Read the model definition and answer for the solid it produces. Units are mm, in the model's axes. A direction names the side the tool comes from. Give positions to 0.01 mm unless a question says otherwise; leave off trailing zeros. Order: outer loops, then holes, each group sorted by start corner. A loop starts at its lowest first (then second) coordinate and runs counter-clockwise, first axis right, second up. Notation, with made-up numbers: M -3.5,-30.5 L 54.5,-30.5 A27 ccw 54.5,-10.5 Z; hole C -25.75,16 d11. An arc over 180 degrees is marked long. One line per item, written item: value. Start each with the question number.
from build123d import *

# Parameters (mm, degrees)
PAD_DEPTH    = 6
POCKET_DEPTH = 5


with BuildPart() as part:
    # Sketch004 → Pad (new body)
    with BuildSketch(Plane.XY):
        with BuildLine():
            Line((-34.247254, 29.142098), (-34.247254, -40.731934))
            ThreePointArc((-34.247254, -40.731934), (-31.611215, -47.095895), (-25.247254, -49.731934))
            Line((-25.247254, -49.731934), (26.073956, -49.731934))
            ThreePointArc((26.073956, -49.731934), (31.73081, -47.388788), (34.073956, -41.731934))
            Line((34.073956, -41.731934), (34.073956, 29.142098))
            ThreePointArc((34.073956, 29.142098), (31.73081, 34.798952), (26.073956, 37.142098))
            Line((26.073956, 37.142098), (-26.247254, 37.142098))
            ThreePointArc((-26.247254, 37.142098), (-31.904109, 34.798952), (-34.247254, 29.142098))
        make_face()
    extrude(amount=PAD_DEPTH)

    # Sketch → Pocket (cut)
    with BuildSketch(Plane.XY.offset(6)):
        with BuildLine():
            ThreePointArc((0.2524, -41.074003), (14.410312, -36.50526), (22.890576, -24.282125))
            ThreePointArc((22.890576, -24.282125), (25.200826, -12.310293), (25.333783, -0.118314))
            ThreePointArc((25.333783, -0.118314), (22.825754, 10.910473), (17.275703, 20.765487))
            ThreePointArc((17.275703, 20.765487), (9.874199, 26.772272), (0.569118, 28.840892))
            ThreePointArc((0.55, 28.840771), (0.559559, 28.840801), (0.569118, 28.840892))
            Line((0.55, 28.840771), (0, 28.840771))
            Line((-0.55, 28.840771), (0, 28.840771))
            ThreePointArc((-0.569118, 28.840892), (-0.559559, 28.840801), (-0.55, 28.840771))
            ThreePointArc((-0.569118, 28.840892), (-9.874199, 26.772272), (-17.275703, 20.765487))
            ThreePointArc((-17.275703, 20.765487), (-22.825754, 10.910473), (-25.333783, -0.118314))
            ThreePointArc((-25.333783, -0.118314), (-25.200826, -12.310293), (-22.890576, -24.282125))
            ThreePointArc((-22.890576, -24.282125), (-14.410312, -36.50526), (-0.2524, -41.074003))
            ThreePointArc((-0.231547, -41.073858), (-0.241974, -41.073894), (-0.2524, -41.074003))
            Line((-0.231547, -41.073858), (0, -41.073858))
            Line((0.231547, -41.073858), (0, -41.073858))
            ThreePointArc((0.2524, -41.074003), (0.241974, -41.073894), (0.231547, -41.073858))
        make_face()
    extrude(amount=-POCKET_DEPTH, mode=Mode.SUBTRACT)


solid = part.part
Q1. Consider probe 1 along Z at (x, y) = (7, -39.5); probe 2 along X at (y, z) = (8, 5.6); probe 3 along Y at (x, z) = (9, 4.05). Determine where each line is inside the solid, lowest interval first.
Q2. Find section B-B, the plane y = -20. Give the vertices of the cut face in (x, z), then the cut area to 3 significant figures.
Q3. Determine the mould class of faces 3 (the cylindrical face through (-31.681, -47.026, 2.958)), 4 (the cylindrical face through (25.183, -12.48, 3.535)), 5 (the flat face through (-34.247, -5, 3)) for opening direction Y: released by +Y, released by -Y, zero draft, split by the parting line, or undercut.
Q4. Each of these flat-tipped pins is pushed along its axis until it touches: pin 1 (15.5 mm diameter, centred on x = 10.5, y = -4.5, fed in from +Z); pin 2 (5 mm diameter, centred on x = 18, y = -17.5, fed in from -Z). Where does it stop, or does it pass through?
Q5. Find section D-D, the plane y = 32. Give the vertices of the cut face in (x, z).
Q6. Find section C-C, the plane x = 2.5. Give the vertices of the cut face in (y, z).
Q7. A tool of negligible diameter and unlimited length cuts with its end or side. For faces 1 (the cylindrical face through (-22.768, 11.059, 3.535)), 2 (the flat face through (-23, 14, 6)), from which of +Z, -Z, +X, -X, +Y, -Y can it reach the whole face along a straight path? Write none if from no direction.
Evaluation:
1. probe 1: 0 to 1
1. probe 2: -34.25 to -23.82, 23.82 to 34.07
1. probe 3: -49.73 to -39.49, 27.17 to 37.14
2. outline: M -34.25,0 L 34.07,0 L 34.07,6 L 23.97,6 L 23.97,1 L -23.97,1 L -23.97,6 L -34.25,6 Z
2. area: 170 mm2
3. face 3: released by -Y
3. face 4: undercut
3. face 5: zero draft
4. pin 1: z = 1
4. pin 2: z = 0
5. outline: M -33.72,0 L 33.55,0 L 33.55,6 L -33.72,6 Z
6. outline: M -49.73,0 L 37.14,0 L 37.14,6 L 28.78,6 L 28.78,1 L -41,1 L -41,6 L -49.73,6 Z
7. face 1: +Z
7. face 2: +Z, +X, -X, +Y, -Y
